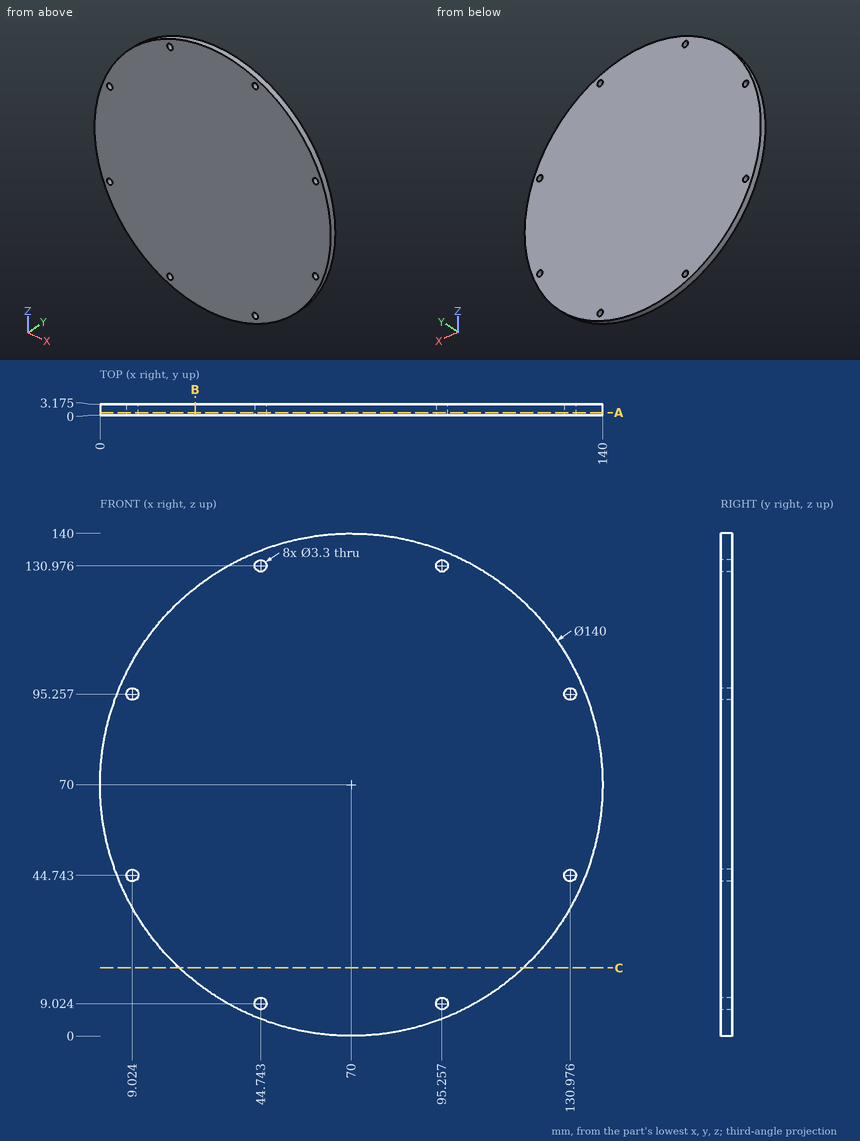
The drawing under review shows one solid part. Ordinate dimensions are in mm from its lowest x, y, z. Round coordinates to 2 decimals unless told otherwise and drop trailing zeros. Write each loop counter-clockwise with the first axis right and the second up, starting at its lowest first coordinate (ties: lowest second). Pieces come first, ordered by that corner, then holes. Notation, with made-up numbers: (22.25, 30.25) - (49.25, 30.25) arc R8 cw to (49.25, 36.25) - close; hole circle Ø3 at (-27, -26). An arc over 180 degrees is marked (long way). Use one line per item in the form item = value.
Q1. Consider section B-B (x = 26.5). State the section outline as (y, z) points (3 decimals).
Answer key:
outline = (0, 15.157) - (3.175, 15.157) - (3.175, 124.843) - (0, 124.843) - close
Q2. Insertion check: pin 1 Ø1.5 at (x, y) = (79, 1) entering from -Z. The pin has a flat end and moves straight along its axis. Give the tip position at first contact, or say it passes through.
Answer key:
pin_1 = 0.49
Q3. For line 1 (Z direction, x = 46, y = 1.9) (1 decimal); line 2 (Z direction, x = 44.5, y = 2.05); line 3 (X direction, y = 2.1, z = 96), list the stretches that pass through material, from the lowest coordinate up. Write a range as [from, to].
Answer key:
line_1 = [4.2, 8], [10.1, 129.9], [132, 135.8]
line_2 = [4.81, 7.39], [10.66, 129.34], [132.61, 135.19]
line_3 = [5.01, 7.55], [10.5, 129.5], [132.45, 134.99]
Q4. Consider section A-A (y = 0.8). State how many separate pieces and enclosed holes the cut face has, and give its area (3 significant figures).
Answer key:
separate_pieces = 1
enclosed_holes = 8
area = 15,300 mm2
Q5. Consider section C-C (z = 19). State the section outline as (x, y) points (3 decimals).
Answer key:
outline = (22.052, 0) - (117.948, 0) - (117.948, 3.175) - (22.052, 3.175) - close
